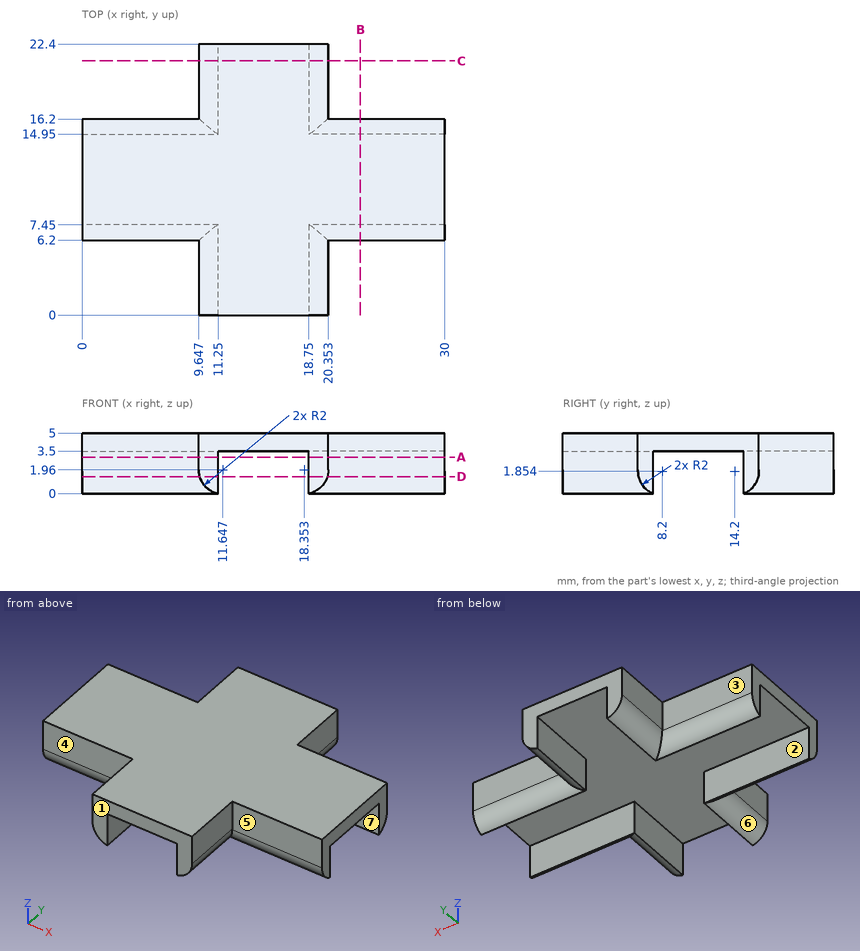
Can you work these out from the drawing? Everything is in mm from the part's minimum corner. A direction names the side the tool comes from. Round coordinates to 2 decimals unless told otherwise and drop trailing zeros. Loops run counter-clockwise (first coordinate to the right, second up) from the corner with the lowest first, then second, coordinate; pieces in that order, holes last. Notation, with made-up numbers: (19, 37.5) -> (70, 37.5) arc R24 cw to (70, 73.5) -> close; hole circle Ø9 at (-30, 86.5). An arc over 180 degrees is marked (long way). One line per question, with ' | ' between items.
(1) If we section it at B-B on x = 23: List the corners of the cut face in (y, z) for me.
Model answer:
outline: (6.2, 1.85) arc R2 ccw to (7.45, 0) -> (7.45, 3.5) -> (14.95, 3.5) -> (14.95, 0) arc R2 ccw to (16.2, 1.85) -> (16.2, 5) -> (6.2, 5) -> close
(2) If I drill on probe 1 along Y at (x, z) = (20.5, 2.5); probe 2 along X at (y, z) = (16, 1.25); probe 3 along X at (y, z) = (20.25, 3.4), over which ranges is the centre line in solid material (lowest first)?
Model answer:
probe 1: y = 6.2 to 7.45, 14.95 to 16.2 | probe 2: x = 0 to 11.25, 18.75 to 30 | probe 3: x = 9.65 to 11.25, 18.75 to 20.35
(3) For pin 1 Ø3 at (y, z) = (3, 2) entering from -X; pin 2 Ø3 at (x, z) = (5, 3.5) entering from +Y; pin 3 Ø6.5 at (x, y) = (19, 11.5) entering from -Z, each with a flat end and sliding along its axis, tell me the tip position at first contact or that it passes through.
Model answer:
pin 1: stops at x = 9.65 | pin 2: stops at y = 16.2 | pin 3: stops at z = 3.5
(4) If we section it at C-C on y = 21: List the corners of the cut face in (x, z) for me.
Model answer:
outline: (9.65, 1.96) arc R2 ccw to (11.25, 0) -> (11.25, 3.5) -> (18.75, 3.5) -> (18.75, 0) arc R2 ccw to (20.35, 1.96) -> (20.35, 5) -> (9.65, 5) -> close
(5) If we section it at D-D on z = 1.4: List the corners of the cut face in (x, y) for me.
Model answer:
outline: (0, 6.25) -> (9.73, 6.25) -> (9.73, 0) -> (11.25, 0) -> (11.25, 7.45) -> (0, 7.45) -> close; (0, 14.95) -> (11.25, 14.95) -> (11.25, 22.4) -> (9.73, 22.4) -> (9.73, 16.15) -> (0, 16.15) -> close; (18.75, 0) -> (20.27, 0) -> (20.27, 6.25) -> (30, 6.25) -> (30, 7.45) -> (18.75, 7.45) -> close; (18.75, 14.95) -> (30, 14.95) -> (30, 16.15) -> (20.27, 16.15) -> (20.27, 22.4) -> (18.75, 22.4) -> close
(6) Thinking about a two-plate mould opening in Y: for the marked faces 1, 2 and 3, which applies, released by +Y, released by -Y, zero draft, split by the parting line, or undercut?
Model answer:
face 1: released by -Y | face 2: undercut | face 3: released by +Y
(7) If we section it at A-A on z = 3: List the corners of the cut face in (x, y) for me.
Model answer:
outline: (0, 6.2) -> (9.65, 6.2) -> (9.65, 0) -> (11.25, 0) -> (11.25, 7.45) -> (0, 7.45) -> close; (0, 14.95) -> (11.25, 14.95) -> (11.25, 22.4) -> (9.65, 22.4) -> (9.65, 16.2) -> (0, 16.2) -> close; (18.75, 0) -> (20.35, 0) -> (20.35, 6.2) -> (30, 6.2) -> (30, 7.45) -> (18.75, 7.45) -> close; (18.75, 14.95) -> (30, 14.95) -> (30, 16.2) -> (20.35, 16.2) -> (20.35, 22.4) -> (18.75, 22.4) -> close
(8) For the marked faces 4, 5, 6 and 7, which set-ups out of +Z, -Z, +X, -X, +Y, -Y let a thin tool reach every point of the face, with its end or its side?
Model answer:
face 4: +Z, -Z, -X, -Y | face 5: +Z, -Z, +X, -Y | face 6: -Z, -X, -Y | face 7: -Z, +X, -X
